from build123d import *

# Parameters (mm, degrees)
BOSS_EXTRUDE1_DEPTH = 30
SKETCH2_R           = 2
CUT_EXTRUDE1_DEPTH  = 3


with BuildPart() as part:
    # Sketch1 → Boss-Extrude1 (new body)
    with BuildSketch(Plane.XY):
        Polygon((0, 0), (0, 20), (3, 20), (3, 3), (15, 3), (15, 0), align=None)
    extrude(amount=BOSS_EXTRUDE1_DEPTH)

    # Sketch2 → Cut-Extrude1 (cut)
    with BuildSketch(Plane(origin=(0, 3, 0), x_dir=(1, 0, 0), z_dir=(0, 1, 0))):
        with Locations(Location((9, -7, 0), (0, 0, 180))):
            Circle(SKETCH2_R)
        with Locations((9, -23)):
            Circle(SKETCH2_R)
    extrude(amount=-CUT_EXTRUDE1_DEPTH, mode=Mode.SUBTRACT)


solid = part.part
Geometry check sheet. Reference: the model listing, model coordinates, mm. A direction names the side the tool comes from. Coordinates: 2 decimals unless noted, no trailing zeros. Write each loop counter-clockwise with the first axis right and the second up, starting at its lowest first coordinate (ties: lowest second). Pieces come first, ordered by that corner, then holes. Notation, with made-up numbers: (63, 19) -> (103, 19) arc R19 cw to (103, 48) -> close; hole circle Ø9 at (-13.75, 47). An arc over 180 degrees is marked (long way). One line per question, with ' | ' between items.
1. Draft check along Z on faces 3 (the flat face through (1, 20, 15)), 4 (the flat face through (2.5, 7.1, 0)), 5 (the cylindrical face through (7.526, 1.521, 21.648)). Enter one of: +Z half, -Z half, draft (parallel to the pull), parting line (faces both ways), or undercut.
Answers:
face 3: draft | face 4: -Z half | face 5: undercut
2. Depth check by flat-ended pin: pin 1 Ø1.5 at (x, z) = (13, 19.5) entering from +Y; pin 2 Ø2 at (y, z) = (11, 18) entering from +X. Enter the tip coordinate at first touch or a pass-through.
Answers:
pin 1: stops at y = 3 | pin 2: stops at x = 3
3. Cross-section at A-A on x = 9. Record the cut outline in (y, z), and give its area (3 significant figures).
Answers:
outline: (0, 0) -> (3, 0) -> (3, 5) -> (0, 5) -> close; (0, 9) -> (3, 9) -> (3, 21) -> (0, 21) -> close; (0, 25) -> (3, 25) -> (3, 30) -> (0, 30) -> close | area: 66.0 mm²
4. Thickness scan on probe 1 along Z at (x, y) = (9, 1.95); probe 2 along X at (y, z) = (2.4, 23); probe 3 along X at (y, z) = (11.75, 27.5). Record the ranges inside material, lowest first. Write a range as from..to.
Answers:
probe 1: z = 0..5, 9..21, 25..30 | probe 2: x = 0..7, 11..15 | probe 3: x = 0..3
5. Cross-section at B-B on z = 23. Record the cut outline in (x, y), and give its area (3 significant figures).
Answers:
outline: (0, 0) -> (7, 0) -> (7, 3) -> (3, 3) -> (3, 20) -> (0, 20) -> close; (11, 0) -> (15, 0) -> (15, 3) -> (11, 3) -> close | area: 84.0 mm²
6. Cross-section at D-D on x = 6.5. Record the cut outline in (y, z), and give its area (3 significant figures).
Answers:
outline: (0, 0) -> (3, 0) -> (3, 30) -> (0, 30) -> close | area: 90.0 mm²
7. Set-up check for faces 1 (the cylindrical face through (9, 2, 9)), 2 (the flat face through (9, 3, 15)): record each of +Z, -Z, +X, -X, +Y, -Y from which the full face is reachable in a straight line by a thin tool's end or side.
Answers:
face 1: +Y, -Y | face 2: +Z, -Z, +X, +Y
8. Cross-section at C-C on z = 17.25. Record the cut outline in (x, y).
Answers:
outline: (0, 0) -> (15, 0) -> (15, 3) -> (3, 3) -> (3, 20) -> (0, 20) -> close
